Study the drawing (mm; zero at the part's minimum x, y, z) and answer. Round coordinates to 2 decimals unless told otherwise and drop trailing zeros. Order: outer loops, then holes, each group sorted by start corner. A loop starts at its lowest first (then second) coordinate and runs counter-clockwise, first axis right, second up. Notation, with made-up numbers: (36, -6.5) - (76, -6.5) arc R19 cw to (76, 13.5) - close; hole circle Ø10 at (34, -21). An arc over 180 degrees is marked (long way). Put each result on its own line as item: value.
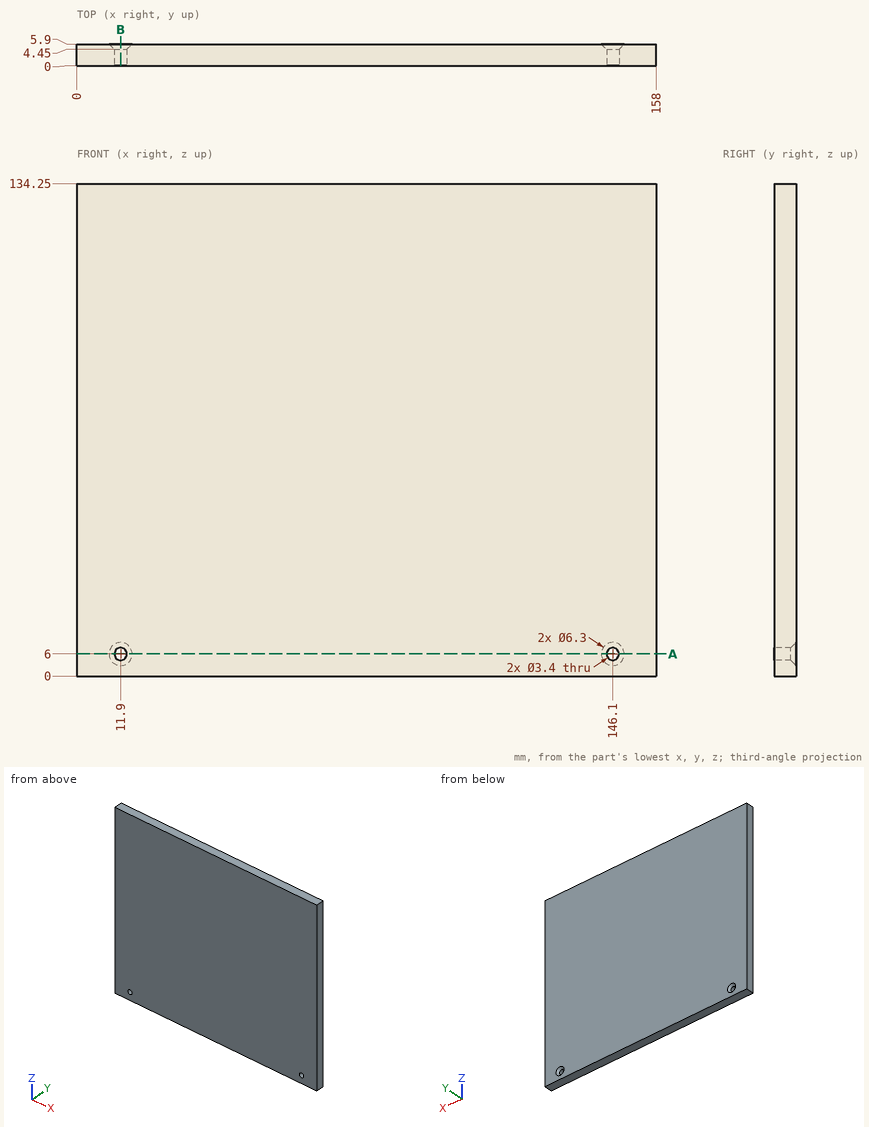
1) Straight lines are drawn through the part: L1, parallel to X at y = 1.8, z = 6; L2, parallel to Z at x = 11.9, y = 2.15. For each, find the intervals that lie inside material, in ascending order. Write a range as from..to.
Findings below:
L1: x = 0..10.2, 13.6..144.4, 147.8..158
L2: z = 0..4.3, 7.7..134.25
2) A cutting plane is placed at A-A on z = 6. Write down the section's boundary in (x, y), then the cut area to 3 significant figures.
Findings below:
outline: (0, 0) - (10.2, 0) - (10.2, 4.45) - (8.75, 5.9) - (0, 5.9) - close; (13.6, 0) - (144.4, 0) - (144.4, 4.45) - (142.95, 5.9) - (15.05, 5.9) - (13.6, 4.45) - close; (147.8, 0) - (158, 0) - (158, 5.9) - (149.25, 5.9) - (147.8, 4.45) - close
area: 888 mm2
3) Given pin 1 Ø3 at (x, z) = (146.1, 6) entering from +Y; pin 2 Ø4 at (x, z) = (11.9, 6) entering from +Y, each flat-ended and moving along its own axis, determine where each tip first touches the part or whether it passes through.
Findings below:
pin 1: passes through
pin 2: stops at y = 4.75
4) A cutting plane is placed at B-B on x = 11.9. Write down the section's boundary in (y, z).
Findings below:
outline: (0, 0) - (5.9, 0) - (5.9, 2.85) - (4.45, 4.3) - (0, 4.3) - close; (0, 7.7) - (4.45, 7.7) - (5.9, 9.15) - (5.9, 134.25) - (0, 134.25) - close
